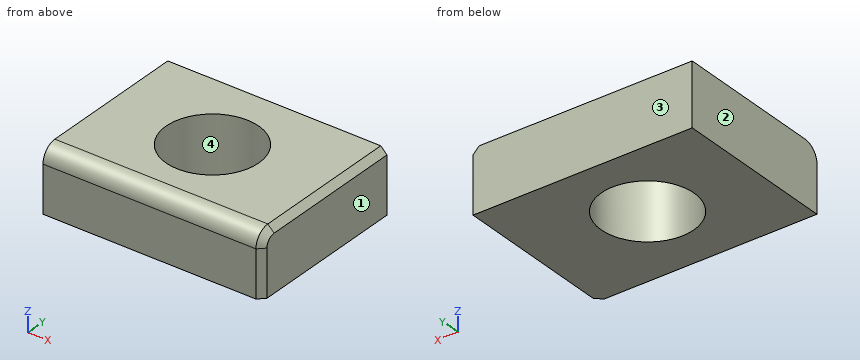
from build123d import *

# Parameters (mm, degrees)
F0_W     = 109.517686
F0_H     = 66.721742
F1_DEPTH = 50.8
F2_R     = 37.612171
F3_DEPTH = 50.801
F4_R     = 12.7
F5_SIZE  = 5.08


with BuildPart() as f1:
    # F0 (on Top) → F1 (new body)
    with BuildSketch(Plane.XY):
        Polygon((177.8, 0), (0, 0), (0, -133.443484), (40.524788, -133.443484), (40.524788, -66.721742), (150.042474, -66.721742), (150.042474, -133.443484), (177.8, -133.443484), align=None)
        with Locations((95.283631, -100.082613)):
            Rectangle(F0_W, F0_H)
    extrude(amount=F1_DEPTH)

    # F2 (on face) → F3 (cut, through all)
    with BuildSketch(Plane.XY.offset(50.8)):
        with Locations((85.144848, -64.497687)):
            Circle(F2_R)
    extrude(amount=-F3_DEPTH, mode=Mode.SUBTRACT)

    # F4
    f4_edges = [f1.edges().sort_by_distance(p)[0] for p in [
        (88.9, -133.443484, 50.8),
    ]]
    fillet(f4_edges, radius=F4_R)

    # F5
    f5_edges = [f1.edges().sort_by_distance(p)[0] for p in [
        (177.8, -60.371742, 50.8),
    ]]
    chamfer(f5_edges, length=F5_SIZE)


solid = f1.part
Source: CAD feature listing. Evaluate the final solid. Frame: model axes, mm. Face numbers are marked on the shaded views. Round coordinates to 2 decimals unless told otherwise and drop trailing zeros. Order: outer loops, then holes, each group sorted by start corner. A loop starts at its lowest first (then second) coordinate and runs counter-clockwise, first axis right, second up. Notation, with made-up numbers: (20, 55.5) - (46, 55.5) arc R12 ccw to (46, 63.5) - close; hole circle Ø9 at (-4, -8). An arc over 180 degrees is marked (long way). Use a Markdown table: item, result. Add a question column.
1. Mould query, pull axis X, two halves, no side actions, for the marked faces 1, 2, 3 and 4. Classes: +X half, -X half, draft (parallel to the pull), parting line (faces both ways), or undercut.
2. Section query B-B (y = -70.5). Return the cut outline in (x, z) (3 decimals), then the cut area to 3 significant figures.
3. Section query A-A (x = 94). Return the cut outline in (y, z), then the cut area to 3 significant figures.
4. Section query C-C (z = 22.5). Return the cut outline in (x, y).
5. Line query: probe 1 along X at (y, z) = (-64, 39); probe 2 along Y at (x, z) = (69, 41); probe 3 along Y at (x, z) = (70, 27.5). Output: solid intervals per line, ascending.
Derived:
| question | item | result |
|---|---|---|
| 1 | face 1 | +X half |
| 1 | face 2 | -X half |
| 1 | face 3 | draft |
| 1 | face 4 | undercut |
| 2 | outline | (0, 0) - (48.015, 0) - (48.015, 50.8) - (0, 50.8) - close; (122.275, 0) - (177.8, 0) - (177.8, 45.72) - (172.72, 50.8) - (122.275, 50.8) - close |
| 2 | area | 5,250 mm2 |
| 3 | outline | (-133.44, 0) - (-101.05, 0) - (-101.05, 50.8) - (-120.74, 50.8) arc R12.7 ccw to (-133.44, 38.1) - close; (-27.94, 0) - (0, 0) - (0, 50.8) - (-27.94, 50.8) - close |
| 3 | area | 3,030 mm2 |
| 4 | outline | (0, -133.44) - (172.72, -133.44) - (177.8, -128.36) - (177.8, 0) - (0, 0) - close; hole circle Ø75.22 at (85.14, -64.5) |
| 5 | probe 1 | 0 to 47.54, 122.75 to 177.8 |
| 5 | probe 2 | -133.11 to -98.47, -30.53 to 0 |
| 5 | probe 3 | -133.44 to -98.93, -30.07 to 0 |
